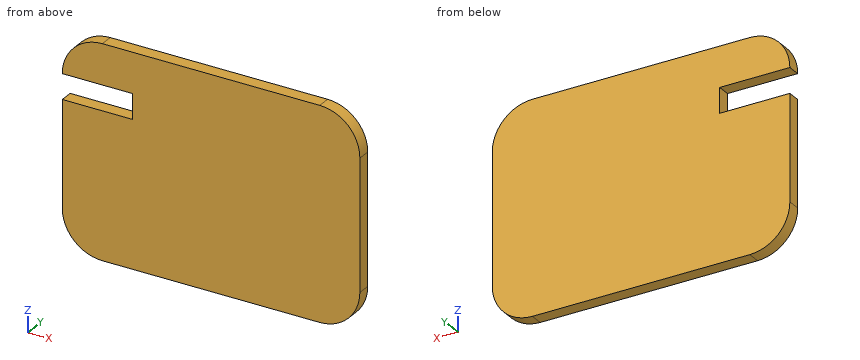
from build123d import *

# Parameters (mm, degrees)
F1_DEPTH = 13
F2_W     = 75
F2_H     = 25
F3_DEPTH = 25


with BuildPart() as f1:
    # F0 (on Front) → F1 (new body)
    with BuildSketch(Plane.XZ):
        with BuildLine():
            Line((145.069164, 99.403447), (-71.930836, 99.403447))
            ThreePointArc((-71.930836, 99.403447), (-100.215108, 87.687718), (-111.930836, 59.403447))
            Line((-111.930836, 59.403447), (-111.930836, -70.596553))
            ThreePointArc((-111.930836, -70.596553), (-100.215108, -98.880824), (-71.930836, -110.596553))
            Line((-71.930836, -110.596553), (145.069164, -110.596553))
            ThreePointArc((145.069164, -110.596553), (173.353435, -98.880824), (185.069164, -70.596553))
            Line((185.069164, -70.596553), (185.069164, 59.403447))
            ThreePointArc((185.069164, 59.403447), (173.353435, 87.687718), (145.069164, 99.403447))
        make_face()
    extrude(amount=F1_DEPTH)

    # F2 (on face) → F3 (cut)
    with BuildSketch(Plane.XZ.offset(13)):
        with Locations((-79.382428, 46.903447)):
            Rectangle(F2_W, F2_H)
    extrude(amount=-F3_DEPTH, mode=Mode.SUBTRACT)


solid = f1.part
Input: part model. Units: mm. Frame: model coordinates. Coordinates: 2 decimals unless noted, no trailing zeros. Loops run counter-clockwise (first coordinate to the right, second up) from the corner with the lowest first, then second, coordinate; pieces in that order, holes last.
Q1. Material intervals for line 1 (Z direction, x = -62, y = -3.5); line 2 (X direction, y = -11.5, z = -72.5); line 3 (X direction, y = -4.75, z = 59), sorted ascending.
Q2. Contact query for a flat-ended pin moving along its axis: pin 1 (6 mm diameter, centred on y = -4, z = 73.5, fed in from +X). Output: stop coordinate, or through.
Q3. Cut plane A-A (y = -2.5). Output: boundary loops of the cut face in (x, z).
Working result:
1. line 1: z = -110.6 to 34.4, 59.4 to 99.4
1. line 2: x = -111.89 to 185.02
1. line 3: x = -41.88 to 185.07
2. pin 1: stops at x = 183.5
3. outline: (-111.93, -70.6) arc R40 ccw to (-71.93, -110.6) - (145.07, -110.6) arc R40 ccw to (185.07, -70.6) - (185.07, 59.4) arc R40 ccw to (145.07, 99.4) - (-71.93, 99.4) arc R40 ccw to (-111.93, 59.4) - (-41.88, 59.4) - (-41.88, 34.4) - (-111.93, 34.4) - close
